The listing builds one solid part. Answer for the finished solid, in the listing's coordinates (mm). Coordinates: 2 decimals unless noted, no trailing zeros. Write each loop counter-clockwise with the first axis right and the second up, starting at its lowest first coordinate (ties: lowest second). Pieces come first, ordered by that corner, then holes.
from build123d import *

# Parameters (mm, degrees)
EXTRUDE_1_DEPTH     = 8
CUT_EXTRUDE_1_DEPTH = 9


with BuildPart() as part:
    # Эскиз1 → Бобышка-Вытянуть1 (new body)
    with BuildSketch(Plane.XY):
        Polygon((0, 0), (0, 8), (35, 8), (39.256106995, 4.595114404), (39.256106995, 0), align=None)
    extrude(amount=EXTRUDE_1_DEPTH)

    # Эскиз2 → Вырез-Вытянуть1 (cut, through all)
    with BuildSketch(Plane.XZ):
        Polygon((32.26555928, 0), (39.256106995, 0), (39.256106995, 8), (38.325183504, 6.338802332), align=None)
    extrude(amount=-CUT_EXTRUDE_1_DEPTH, mode=Mode.SUBTRACT)


solid = part.part
Q1. The part is cut by section A-A, the plane y = 6. Write down the section's boundary in (x, z).
Answers below:
outline: (0, 0) - (32.27, 0) - (37.5, 5.48) - (37.5, 8) - (0, 8) - close
Q2. The part is cut by section B-B, the plane z = 4.75. Write down the section's boundary in (x, y), then the cut area to 3 significant figures.
Answers below:
outline: (0, 0) - (36.81, 0) - (36.81, 6.55) - (35, 8) - (0, 8) - close
area: 293 mm2
Q3. Find the intervals of material crossed by probe 1 along X at (y, z) = (7.5, 4.5) (3 decimals); probe 2 along X at (y, z) = (0.75, 7); probe 3 along Z at (x, y) = (37.5, 2.25), in increasing order.
Answers below:
probe 1: x = 0 to 35.625
probe 2: x = 0 to 38.7
probe 3: z = 5.48 to 8
Q4. Given pin 1 (1 mm diameter, centred on y = 2, z = 6.5, fed in from +X); pin 2 (1 mm diameter, centred on y = 3.5, z = 2, fed in from +X), each flat-ended and moving along its own axis, determine where each tip first touches the part or whether it passes through.
Answers below:
pin 1: stops at x = 38.7
pin 2: stops at x = 34.66
